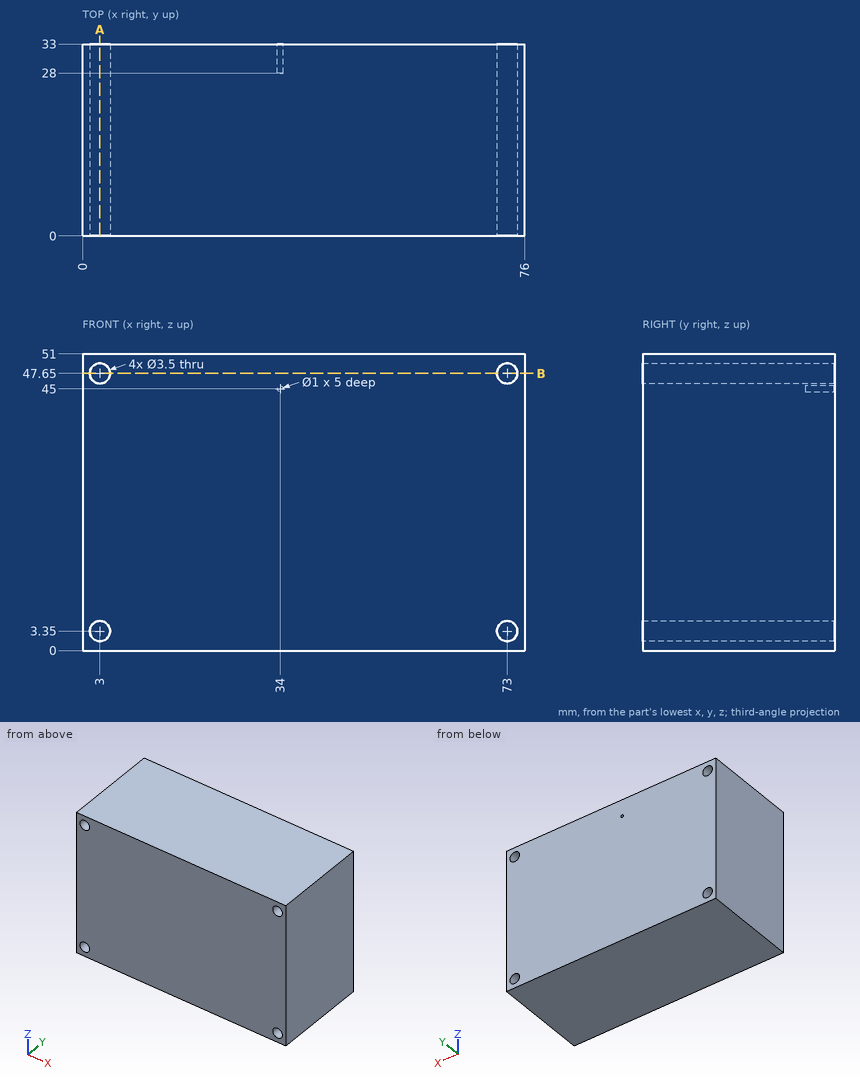
Answer from the drawing. Dimensions are ordinates in mm from the lowest x, y and z of the part. Coordinates: 2 decimals unless noted, no trailing zeros. Write each loop counter-clockwise with the first axis right and the second up, starting at its lowest first coordinate (ties: lowest second). Pieces come first, ordered by that corner, then holes. Notation, with made-up numbers: M 60,54 L 90,54 A14 cw 90,60 Z; hole C 7.25,-14.75 d6. An arc over 180 degrees is marked long. Write item = value, one per line.
1. Flat-ended cylindrical pins translate along their axes: pin 1 (4 mm diameter, centred on x = 73, z = 3.35, fed in from +Y); pin 2 (0.8 mm diameter, centred on x = 34, z = 45, fed in from +Y). Find the tip coordinate at first contact, or state that the pin passes through.
Solution:
pin_1 = 33
pin_2 = 28
2. The part is cut by section A-A (x = 3). Determine the outline of the cut face in (y, z), then the cut area to 3 significant figures.
Solution:
outline = M 0,0 L 33,0 L 33,1.6 L 0,1.6 Z; M 0,5.1 L 33,5.1 L 33,45.9 L 0,45.9 Z; M 0,49.4 L 33,49.4 L 33,51 L 0,51 Z
area = 1,450 mm2
3. The part is cut by section B-B (z = 47.65). Determine the outline of the cut face in (x, y), then the cut area to 3 significant figures.
Solution:
outline = M 0,0 L 1.25,0 L 1.25,33 L 0,33 Z; M 4.75,0 L 71.25,0 L 71.25,33 L 4.75,33 Z; M 74.75,0 L 76,0 L 76,33 L 74.75,33 Z
area = 2,280 mm2
4. Straight lines are drawn through the part: line 1 (X direction, y = 8, z = 47.65); line 2 (Z direction, x = 73, y = 26); line 3 (Z direction, x = 34, y = 30.85). For each, find the intervals that lie inside material, in ascending order. Write a range as from..to.
Solution:
line_1 = 0..1.25, 4.75..71.25, 74.75..76
line_2 = 0..1.6, 5.1..45.9, 49.4..51
line_3 = 0..44.5, 45.5..51
